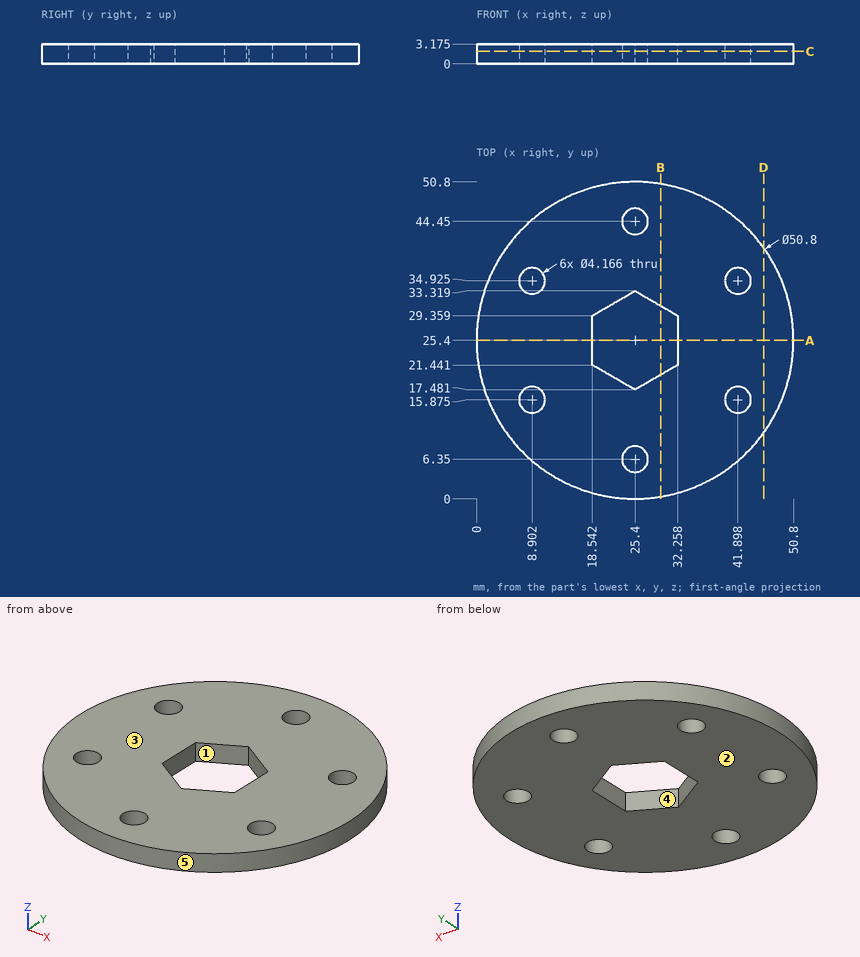
Design review of the part shown in the three views and the two pictorial views. Dimensions are in mm from the part's minimum x, y and z. A direction names the side the tool comes from. Give positions to 0.01 mm unless a question says otherwise; leave off trailing zeros. Loops run counter-clockwise (first coordinate to the right, second up) from the corner with the lowest first, then second, coordinate; pieces in that order, holes last. Notation, with made-up numbers: (79, -40) -> (102, -40) arc R26 cw to (102, -25) -> close; hole circle Ø8 at (41, 13.25). An arc over 180 degrees is marked (long way). Write each question's results on one line, items separated by ' | '.
Q1. Take a section at B-B, the plane x = 29.5. Write out the cut boundary in (y, z) (1 decimal), plus the area to 3 significant figures.
Reply:
outline: (0.3, 0) -> (19.8, 0) -> (19.8, 3.2) -> (0.3, 3.2) -> close; (31, 0) -> (50.5, 0) -> (50.5, 3.2) -> (31, 3.2) -> close | area: 124 mm²
Q2. The part is to be moulded in two halves that separate along X. For the marked faces 3, 4 and 5, say which applies: +X half, -X half, draft (parallel to the pull), parting line (faces both ways), or undercut.
Reply:
face 3: draft | face 4: undercut | face 5: parting line
Q3. Take a section at D-D, the plane x = 46. Write out the cut boundary in (y, z) (1 decimal).
Reply:
outline: (10.5, 0) -> (40.3, 0) -> (40.3, 3.2) -> (10.5, 3.2) -> close
Q4. Take a section at C-C, the plane z = 2. Give the number of separate pieces and of enclosed holes in the cut face, plus the area to 3 significant figures.
Reply:
separate pieces: 1 | enclosed holes: 7 | area: 1,780 mm²
Q5. For pin 1 Ø1.5 at (y, z) = (20.5, 1.5) entering from +X; pin 2 Ø1 at (x, z) = (7.5, 1.5) entering from -Y (1 decimal), all flat-tipped, find the tip position at first contact; note any pin that passes through.
Reply:
pin 1: stops at x = 50.46 | pin 2: stops at y = 6.9
Q6. Wall thickness on L1, parallel to Y at x = 25.4, z = 1.25; L2, parallel to X at y = 15, z = 1.4 (1 decimal); L3, parallel to Y at x = 40, z = 0.4 (1 decimal): over which ranges is each line inside the solid? List them lowest first.
Reply:
L1: y = 0 to 4.27, 8.43 to 17.48, 33.32 to 42.37, 46.53 to 50.8 | L2: x = 2.2 to 7, 10.8 to 40, 43.8 to 48.6 | L3: y = 4.6 to 15, 16.7 to 34.1, 35.8 to 46.2
Q7. Take a section at A-A, the plane y = 25.4. Write out the cut boundary in (x, z) (1 decimal).
Reply:
outline: (0, 0) -> (18.5, 0) -> (18.5, 3.2) -> (0, 3.2) -> close; (32.3, 0) -> (50.8, 0) -> (50.8, 3.2) -> (32.3, 3.2) -> close
Q8. Machinability: for the marked faces 1 and 2, which of the approach directions +Z, -Z, +X, -X, +Y, -Y give a long, thin tool a straight path to every point of the face, cutting with its end or side? Answer none if there is none.
Reply:
face 1: +Z, -Z | face 2: -Z, +X, -X, +Y, -Y
